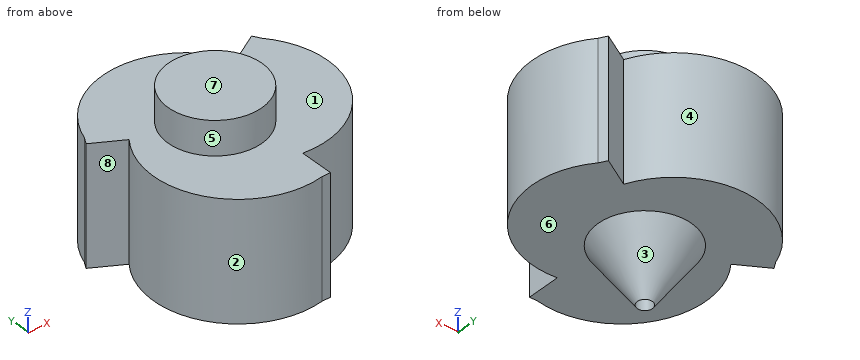
```python
from build123d import *

# Parameters (mm, degrees)
SALIENTE_EXTRUIR1_DEPTH = 18
SALIENTE_EXTRUIR2_START = 1.5
CROQUIS2_R              = 2.7
SALIENTE_EXTRUIR2_DEPTH = 1.5
SALIENTE_EXTRUIR3_DEPTH = 1.5
CROQUIS6_W              = 5.4
CROQUIS6_H              = 1.803822617
SALIENTE_EXTRUIR7_DEPTH = 10
CROQUIS10_W             = 5.4
CROQUIS10_H             = 10
CORTAR_EXTRUIR3_DEPTH   = 10
CROQUIS11_W             = 8.35
CROQUIS11_H             = 6


with BuildPart() as part:
    # Croquis1 → Saliente-Extruir1 (new body)
    with BuildSketch(Plane.XY):
        with BuildLine():
            Line((-53.667784589, 33.4650382), (-54.417784589, 34.764076306))
            Line((-54.417784589, 34.764076306), (-59.613937012, 31.764076306))
            ThreePointArc((-59.613937012, 31.764076306), (-73.945502317, 40.827707086), (-87.584573208, 30.752047693))
            Line((-87.584573208, 30.752047693), (-88.334573208, 29.453009587))
            Line((-88.334573208, 29.453009587), (-83.138420786, 26.453009587))
            ThreePointArc((-83.138420786, 26.453009587), (-83.82197264, 9.509694567), (-68.276660199, 2.735742387))
            Line((-68.276660199, 2.735742387), (-66.776660199, 2.735742387))
            Line((-66.776660199, 2.735742387), (-66.776660199, 8.735742387))
            ThreePointArc((-66.776660199, 8.735742387), (-51.761543041, 16.615426627), (-53.667784589, 33.4650382))
        make_face()
        with BuildLine():
            Line((-54.507549641, 31.745180452), (-55.016343575, 32.626437397))
            Line((-55.016343575, 32.626437397), (-60.212495998, 29.626437397))
            ThreePointArc((-60.212495998, 29.626437397), (-72.508207296, 39.071771198), (-85.675250182, 30.884718699))
            Line((-85.675250182, 30.884718699), (-86.184044116, 30.003461754))
            Line((-86.184044116, 30.003461754), (-80.987891693, 27.003461754))
            ThreePointArc((-80.987891693, 27.003461754), (-83.019935064, 11.632396511), (-69.346218174, 4.322929129))
            Line((-69.346218174, 4.322929129), (-68.328630306, 4.322929129))
            Line((-68.328630306, 4.322929129), (-68.328630306, 10.322929129))
            ThreePointArc((-68.328630306, 10.322929129), (-54.000875637, 16.248660571), (-54.507549641, 31.745180452))
        make_face(mode=Mode.SUBTRACT)
    extrude(amount=SALIENTE_EXTRUIR1_DEPTH)

    # Croquis2 → Saliente-Extruir2 (add)
    with BuildSketch(Plane(origin=(0, 0, 0), x_dir=(-1, 0, 0), z_dir=(0, 0, -1)).offset(SALIENTE_EXTRUIR2_START)):
        with BuildLine():
            Line((87.584573208, 30.752047693), (88.334573208, 29.453009587))
            Line((88.334573208, 29.453009587), (83.138420786, 26.453009587))
            ThreePointArc((83.138420786, 26.453009587), (83.82197264, 9.509694567), (68.276660199, 2.735742387))
            Line((68.276660199, 2.735742387), (66.776660199, 2.735742387))
            Line((66.776660199, 2.735742387), (66.776660199, 8.735742387))
            ThreePointArc((66.776660199, 8.735742387), (51.761543041, 16.615426627), (53.667784589, 33.4650382))
            Line((53.667784589, 33.4650382), (54.417784589, 34.764076306))
            Line((54.417784589, 34.764076306), (59.613937012, 31.764076306))
            ThreePointArc((59.613937012, 31.764076306), (73.945502317, 40.827707086), (87.584573208, 30.752047693))
        make_face()
        with Locations((69.843005999, 22.317609427)):
            Circle(CROQUIS2_R, mode=Mode.SUBTRACT)
    extrude(amount=-SALIENTE_EXTRUIR2_DEPTH)

    # Croquis3 → Saliente-Extruir3 (add)
    with BuildSketch(Plane.XY.offset(18)):
        with BuildLine():
            Line((-66.776660199, 8.735742387), (-66.776660199, 2.735742387))
            Line((-66.776660199, 2.735742387), (-68.276660199, 2.735742387))
            ThreePointArc((-68.276660199, 2.735742387), (-83.82197264, 9.509694567), (-83.138420786, 26.453009587))
            Line((-83.138420786, 26.453009587), (-88.334573208, 29.453009587))
            Line((-88.334573208, 29.453009587), (-87.584573208, 30.752047693))
            ThreePointArc((-87.584573208, 30.752047693), (-73.945502317, 40.827707086), (-59.613937012, 31.764076306))
            Line((-59.613937012, 31.764076306), (-54.417784589, 34.764076306))
            Line((-54.417784589, 34.764076306), (-53.667784589, 33.4650382))
            ThreePointArc((-53.667784589, 33.4650382), (-51.761543041, 16.615426627), (-66.776660199, 8.735742387))
        make_face()
    extrude(amount=SALIENTE_EXTRUIR3_DEPTH)

    # Croquis6 → Saliente-Extruir7 (add)
    with BuildSketch(Plane(origin=(0, 0, -1.5), x_dir=(-1, 0, 0), z_dir=(0, 0, -1))):
        with Locations((69.843005999, 21.415698119)):
            Rectangle(CROQUIS6_W, CROQUIS6_H)
    extrude(amount=SALIENTE_EXTRUIR7_DEPTH)

    # Croquis10 → Cortar-Extruir3 (cut)
    with BuildSketch(Plane(origin=(0, 22.317609427, 0), x_dir=(1, 0, 0), z_dir=(0, 1, 0))):
        with Locations((-69.843005999, 6.5)):
            Rectangle(CROQUIS10_W, CROQUIS10_H)
    extrude(amount=-CORTAR_EXTRUIR3_DEPTH, mode=Mode.SUBTRACT)

    # Croquis11 → Revolución1 (revolve)
    with BuildSketch(Plane(origin=(0, 22.317609427, 0), x_dir=(1, 0, 0), z_dir=(0, 1, 0)), mode=Mode.PRIVATE) as revoluci_n1_sk:
        Polygon((-72.543005999, 1.5), (-79.543005999, 1.5), (-72.543005999, 11.5), align=None)
        with Locations((-75.368005999, -22.5)):
            Rectangle(CROQUIS11_W, CROQUIS11_H)
    revolve(revoluci_n1_sk.sketch.rotate(Axis((-71.193005999, 22.317609427, 25.5), (0, 0, -1)), 180), axis=Axis((-71.193005999, 22.317609427, 25.5), (0, 0, -1)))


solid = part.part
```
Input: part model. Units: mm. Frame: model coordinates. Face numbers are marked on the shaded views. A direction names the side the tool comes from. Give positions to 0.01 mm unless a question says otherwise; leave off trailing zeros. Order: outer loops, then holes, each group sorted by start corner. A loop starts at its lowest first (then second) coordinate and runs counter-clockwise, first axis right, second up. Notation, with made-up numbers: M 85,23 L 97,23 A23 cw 97,46 Z; hole C 75.25,24.25 d1. An arc over 180 degrees is marked long. Return JSON: item names as keys, results as strings.
Item 1: Pull-direction query (Y, two-part tool) for the marked faces 1, 2, 3 and 4; classes: +Y half, -Y half, draft (parallel to the pull), parting line (faces both ways), or undercut.
Solutions:
{"face 1": "draft", "face 2": "undercut", "face 3": "parting line", "face 4": "+Y half"}
Item 2: Cut plane C-C (z = 20.5). Return loops of the section in (x, y), then the cut area to 3 significant figures.
Solutions:
{"outline": "C -71.19,22.32 d16.7", "area": "219 mm^2"}
Item 3: First-contact query: P1, Ø5, axis at y = 34.5, z = 16, coming from the +X side; P2, Ø12, axis at x = -80.5, z = 2.5, coming from the +Y side; P3, Ø3, axis at x = -61.5, z = 6, coming from the -Y side. Flat tips, straight axial feed; report the tip coordinate or a pass-through.
Solutions:
{"P1": "x = -52.55", "P2": "y = 40.8", "P3": "y = 8.77"}
Item 4: Ray query, probe 1 along Z at (x, y) = (-59.5, 13); probe 2 along Y at (x, z) = (-82, 5.5); probe 3 along Y at (x, z) = (-81.5, 14). Return the intervals inside material, ascending.
Solutions:
{"probe 1": "-1.5 to 0, 18 to 19.5", "probe 2": "7.16 to 9.96, 25.75 to 27.59, 35.85 to 38.13", "probe 3": "6.65 to 9.3, 26.41 to 27.3, 36.25 to 38.47"}
Item 5: Access query for the marked faces 5, 6, 7 and 8. Directions: +Z, -Z, +X, -X, +Y, -Y. A direction counts if a zero-diameter tool reaches every point of the face in a straight line with its end or side. Return the directions, or none.
Solutions:
{"face 5": "+Z", "face 6": "-Z", "face 7": "+Z, +X, -X, +Y, -Y", "face 8": "+Z, -Z, -X"}
Item 6: Cut plane A-A (z = 6.5). Return loops of the section in (x, y), then the cut area to 3 significant figures.
Solutions:
{"outline": "M -88.33,29.45 L -83.14,26.45 A15.01 ccw -68.28,2.74 L -66.78,2.74 L -66.78,8.74 A15.01 ccw -53.67,33.47 L -54.42,34.76 L -59.61,31.76 A15.01 ccw -87.58,30.75 Z; hole M -86.18,30 L -80.99,27 A13.62 ccw -69.35,4.32 L -68.33,4.32 L -68.33,10.32 A13.62 ccw -54.51,31.75 L -55.02,32.63 L -60.21,29.63 A13.62 ccw -85.68,30.88 Z", "area": "207 mm^2"}
Item 7: Cut plane B-B (x = -57). Return loops of the section in (y, z).
Solutions:
{"outline": "M 10.96,-1.5 L 33.27,-1.5 L 33.27,19.5 L 10.96,19.5 Z; hole M 12.95,0 L 31.48,0 L 31.48,18 L 12.95,18 Z"}
Item 8: Cut plane D-D (z = -7). Return loops of the section in (x, y), then the cut area to 3 significant figures.
Solutions:
{"outline": "C -71.19,22.32 d9; hole C -71.19,22.32 d2.7", "area": "57.9 mm^2"}
